Work out the finished part from the listing and answer in its coordinate system (mm). A direction names the side the tool comes from. Coordinates: 2 decimals unless noted, no trailing zeros. Answer as a JSON object with one key per item and string values. Group by question number.
1) A tool of negligible diameter and unlimited length cuts with its end or side. For faces 1 (the face through (0, 0, 0)), 2 (the face through (12, 0.794, 13)), 3 (the face through (12, -0.794, 13)), from which of +Z, -Z, +X, -X, +Y, -Y can it reach the whole face along a straight path? Write none if from no direction.
2) Each of these flat-tipped pins is pushed along its axis until it touches: P1, Ø6, axis at x = 19, z = 4.5, coming from the -Y side; P2, Ø2, axis at x = 7.5, z = 9, coming from the +Y side; P3, Ø14, axis at x = 8.5, z = 8, coming from the +Y side. Where does it stop, or does it pass through?
3) Find the intervals of material crossed by line 1 along Y through (x, z) = (12, 4); line 2 along Z through (x, y) = (15.5, 0.1); line 3 along X through (y, z) = (-1.4, 12.25), in increasing order.
from build123d import *

# Parameters (mm, degrees)
F1_DEPTH = 25.4
F2_R     = 0.79374


# Not quite as in the source:
# - a fillet or chamfer is up to 0.001 mm smaller than in the source, because OpenCascade refuses the exact size
# - a feature names something its author has since deleted; it is built from what else it names


with BuildPart() as f1:
    # F0 (on Top) → F1 (new body)
    with BuildSketch(Plane.XY):
        with BuildLine():
            ThreePointArc((2.2450640303, -0.79375), (2.3469565702, -0.4026740868), (2.38125, 0))
            ThreePointArc((2.38125, 0), (2.3469565702, 0.4026740868), (2.2450640303, 0.79375))
            ThreePointArc((2.2450640303, 0.79375), (-2.38125, 0), (2.2450640303, -0.79375))
        make_face()
        with BuildLine():
            ThreePointArc((2.2450640303, 0.79375), (2.3469565702, 0.4026740868), (2.38125, 0))
            ThreePointArc((2.38125, 0), (2.3469565702, -0.4026740868), (2.2450640303, -0.79375))
            Line((2.2450640303, -0.79375), (21.2950640303, -0.79375))
            Line((21.2950640303, -0.79375), (21.2950640303, 0))
            Line((21.2950640303, 0), (21.2950640303, 0.79375))
            Line((21.2950640303, 0.79375), (2.2450640303, 0.79375))
        make_face()
    extrude(amount=F1_DEPTH)

    # F2 (radius 0.79375 in the source; OpenCascade refuses exactly that, so slightly less here)
    f2_edges = [f1.edges().sort_by_distance(p)[0] for p in [
        (-2.38125, 0, 25.4),
        (11.770064, -0.79375, 25.4),
        (21.295064, 0, 25.4),
        (11.770064, 0.79375, 25.4),
        (-2.38125, 0, 0),
        (11.770064, -0.79375, 0),
        (21.295064, 0, 0),
        (11.770064, 0.79375, 0),
        (21.295064, 0.79375, 12.7),
        (2.245064, 0.79375, 12.7),
        (2.245064, -0.79375, 12.7),
        (21.295064, -0.79375, 12.7),
    ]]
    fillet(f2_edges, radius=F2_R)


solid = f1.part
Report:
{
 "1": {"face 1": "-Z, +X, -X, +Y, -Y", "face 2": "+Z, -Z, +X, +Y", "face 3": "+Z, -Z, +X, -Y"},
 "2": {"P1": "stops at y = -0.79", "P2": "stops at y = 0.79", "P3": "stops at y = 1.85"},
 "3": {"line 1": "y = -0.79 to 0.79", "line 2": "z = 0.01 to 25.39", "line 3": "x = -1.93 to 1.93"}
}
